The listing builds one solid part. Answer for the finished solid, in the listing's coordinates (mm). Coordinates: 2 decimals unless noted, no trailing zeros. Write each loop counter-clockwise with the first axis right and the second up, starting at its lowest first coordinate (ties: lowest second). Pieces come first, ordered by that corner, then holes.
(1) The part is cut by section B-B on x = 1.2. Give the number of separate pieces and of enclosed holes in the cut face, plus the area to 3 significant figures.
(2) Given P1, Ø1.6, axis at x = 1.5, y = 82, coming from the -Z side (3 decimals); P2, Ø1, axis at x = 2, z = -20, coming from the -Y side; P3, Ø1.6, axis at x = 1.5, z = -8.5, coming from the -Y side; P4, Ø10, axis at y = -4, z = 8.5, coming from the -X side (3 decimals), each flat-ended and moving along its own axis, determine where each tip first touches the part or whether it passes through.
(3) The part is cut by section A-A on z = 55.5. Determine the outline of the cut face in (x, y) (3 decimals).
(4) The part is cut by section C-C on z = 31. Determine the outline of the cut face in (x, y) (3 decimals), plus the area to 3 significant figures.
(5) Straight lines are drawn through the part: line 1 (Z direction, x = 1.3, y = 152.4) (3 decimals); line 2 (Z direction, x = 0.75, y = 229) (3 decimals); line 3 (Y direction, x = 2.65, z = 82). For each, find the intervals that lie inside material, in ascending order.
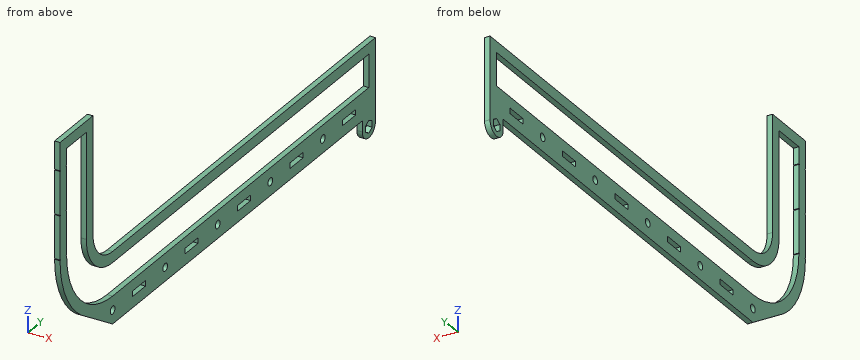
from build123d import *

# Parameters (mm, degrees)
SKETCH2_R           = 2.2606
SKETCH2_W           = 3.175
SKETCH2_H           = 12.7
BOSS_EXTRUDE1_DEPTH = 3.175


with BuildPart() as part:
    # Sketch2 → Boss-Extrude1 (new body)
    with BuildSketch(Plane(origin=(0, 0, 0), x_dir=(0, 0, -1), z_dir=(1, 0, 0))):
        with BuildLine():
            Line((15.875, 254), (22.225, 254))
            ThreePointArc((22.225, 254), (28.575, 247.65), (22.225, 241.3))
            Line((22.225, 241.3), (15.875, 241.3))
            Line((15.875, 241.3), (15.875, 0))
            Line((15.875, 0), (0, -24.593444248))
            ThreePointArc((0, -24.593444248), (-18.649873719, -43.760638523), (-44.45, -50.8))
            Line((-44.45, -50.8), (-44.45, -50.292))
            Line((-44.45, -50.292), (-44.958, -50.292))
            Line((-44.958, -50.292), (-44.958, -50.8))
            Line((-44.958, -50.8), (-69.85, -50.8))
            Line((-69.85, -50.8), (-69.85, -50.292))
            Line((-69.85, -50.292), (-70.358, -50.292))
            Line((-70.358, -50.292), (-70.358, -50.8))
            Line((-70.358, -50.8), (-95.25, -50.8))
            Line((-95.25, -50.8), (-95.25, -50.292))
            Line((-95.25, -50.292), (-95.758, -50.292))
            Line((-95.758, -50.292), (-95.758, -50.8))
            Line((-95.758, -50.8), (-111.76, -50.8))
            Line((-111.76, -50.8), (-111.76, -44.45))
            Line((-111.76, -44.45), (-111.76, -25.4))
            Line((-111.76, -25.4), (-111.76, -19.05))
            Line((-111.76, -19.05), (-44.45, -19.05))
            ThreePointArc((-44.45, -19.05), (-30.979615818, -13.470384182), (-25.4, 0))
            Line((-25.4, 0), (-25.4, 247.65))
            Line((-25.4, 247.65), (-25.4, 254))
            Line((-25.4, 254), (0, 254))
            Line((0, 254), (15.875, 254))
        make_face()
        with Locations((7.9375, 0)):
            Circle(SKETCH2_R, mode=Mode.SUBTRACT)
        with Locations((7.9375, 50.8)):
            Circle(SKETCH2_R, mode=Mode.SUBTRACT)
        with Locations((7.9375, 101.6)):
            Circle(SKETCH2_R, mode=Mode.SUBTRACT)
        with Locations((7.9375, 152.4)):
            Circle(SKETCH2_R, mode=Mode.SUBTRACT)
        with Locations((7.9375, 203.2)):
            Circle(SKETCH2_R, mode=Mode.SUBTRACT)
        with BuildLine():
            Line((-44.958, -44.45), (-69.85, -44.45))
            Line((-69.85, -44.45), (-69.85, -44.958))
            Line((-69.85, -44.958), (-70.358, -44.958))
            Line((-70.358, -44.958), (-70.358, -44.45))
            Line((-70.358, -44.45), (-95.25, -44.45))
            Line((-95.25, -44.45), (-95.25, -44.958))
            Line((-95.25, -44.958), (-95.758, -44.958))
            Line((-95.758, -44.958), (-95.758, -44.45))
            Line((-95.758, -44.45), (-105.41, -44.45))
            Line((-105.41, -44.45), (-105.41, -25.4))
            Line((-105.41, -25.4), (-44.45, -25.4))
            ThreePointArc((-44.45, -25.4), (-26.489487758, -17.960512242), (-19.05, 0))
            Line((-19.05, 0), (-19.05, 247.65))
            Line((-19.05, 247.65), (0, 247.65))
            Line((0, 247.65), (0, 0))
            ThreePointArc((0, 0), (-13.019103576, -31.430896424), (-44.45, -44.45))
            Line((-44.45, -44.45), (-44.45, -44.958))
            Line((-44.45, -44.958), (-44.958, -44.958))
            Line((-44.958, -44.958), (-44.958, -44.45))
        make_face(mode=Mode.SUBTRACT)
        with Locations((7.9375, 228.6)):
            Rectangle(SKETCH2_W, SKETCH2_H, mode=Mode.SUBTRACT)
        with Locations((7.9375, 177.8)):
            Rectangle(SKETCH2_W, SKETCH2_H, mode=Mode.SUBTRACT)
        with Locations((7.9375, 76.2)):
            Rectangle(SKETCH2_W, SKETCH2_H, mode=Mode.SUBTRACT)
        with Locations((7.9375, 127)):
            Rectangle(SKETCH2_W, SKETCH2_H, mode=Mode.SUBTRACT)
        with Locations((7.9375, 25.4)):
            Rectangle(SKETCH2_W, SKETCH2_H, mode=Mode.SUBTRACT)
        Polygon((25.8826, 247.65), (24.0538, 250.825), (20.3962, 250.825), (18.5674, 247.65), (20.3962, 244.505584275), (24.0538, 244.505584275), align=None, mode=Mode.SUBTRACT)
    extrude(amount=BOSS_EXTRUDE1_DEPTH)


solid = part.part
Model answer:
1. separate pieces: 1
1. enclosed holes: 12
1. area: 7,350 mm2
2. P1: stops at z = -15.875
2. P2: stops at y = 241.3
2. P3: stops at y = -12.66
2. P4: passes through
3. outline: (0, -50.8) - (3.175, -50.8) - (3.175, -44.45) - (0, -44.45) - close; (0, -25.4) - (3.175, -25.4) - (3.175, -19.05) - (0, -19.05) - close
4. outline: (0, -48.987) - (3.175, -48.987) - (3.175, -42.366) - (0, -42.366) - close; (0, -21.547) - (3.175, -21.547) - (3.175, -13.491) - (0, -13.491) - close
4. area: 46.6 mm2
5. line 1: z = -15.875 to -10.198, -5.677 to 0, 19.05 to 25.4
5. line 2: z = -15.875 to -9.525, -6.35 to 0, 19.05 to 25.4
5. line 3: y = -50.8 to -44.45, -25.4 to -19.05
